from build123d import *

# Parameters (mm, degrees)
SKETCH_1_W      = 2
SKETCH_1_H      = 5
EXTRUDE_1_DEPTH = 2
FILLET_1_R      = 10


with BuildPart() as part:
    # 草图1 → 凸台-拉伸1 (new body)
    with BuildSketch(Plane(origin=(0, 0, 0), x_dir=(1, 0, 0), z_dir=(0, 1, 0))):
        with BuildLine():
            Line((10, 0), (0, 0))
            Line((0, 0), (0, -5))
            Line((0, -5), (0, -13.5))
            ThreePointArc((0, -13.5), (1.060660172, -13.939339828), (1.5, -15))
            ThreePointArc((1.5, -15), (1.060660172, -16.060660172), (0, -16.5))
            Line((0, -16.5), (0, -43.5))
            ThreePointArc((0, -43.5), (1.060660172, -43.939339828), (1.5, -45))
            ThreePointArc((1.5, -45), (1.060660172, -46.060660172), (0, -46.5))
            Line((0, -46.5), (0, -73.5))
            ThreePointArc((0, -73.5), (1.060660172, -73.939339828), (1.5, -75))
            Line((1.5, -75), (2.5, -75))
            Line((2.5, -75), (2.5, -72.5))
            Line((2.5, -72.5), (7.5, -72.5))
            Line((7.5, -72.5), (7.5, -75))
            Line((7.5, -75), (8.5, -75))
            ThreePointArc((8.5, -75), (8.939339828, -73.939339828), (10, -73.5))
            Line((10, -73.5), (10, -46.5))
            ThreePointArc((10, -46.5), (8.5, -45), (10, -43.5))
            Line((10, -43.5), (10, -16.5))
            ThreePointArc((10, -16.5), (8.5, -15), (10, -13.5))
            Line((10, -13.5), (10, -5))
            Line((10, -5), (10, 0))
        make_face()
        Polygon((2.5, -72.5), (2.5, -75), (5, -75), (7.5, -75), (7.5, -72.5), align=None)
        Polygon((5, -75), (2.5, -75), (2.5, -77.5), (7.5, -77.5), (7.5, -75), align=None)
        with BuildLine():
            Line((2.5, -75), (1.5, -75))
            ThreePointArc((1.5, -75), (1.060660172, -76.060660172), (0, -76.5))
            Line((0, -76.5), (0, -103.5))
            ThreePointArc((0, -103.5), (1.060660172, -103.939339828), (1.5, -105))
            ThreePointArc((1.5, -105), (1.060660172, -106.060660172), (0, -106.5))
            Line((0, -106.5), (0, -133.5))
            ThreePointArc((0, -133.5), (1.060660172, -133.939339828), (1.5, -135))
            ThreePointArc((1.5, -135), (1.060660172, -136.060660172), (0, -136.5))
            Line((0, -136.5), (0, -145))
            Line((0, -145), (0, -150))
            Line((0, -150), (10, -150))
            Line((10, -150), (10, -145))
            Line((10, -145), (10, -136.5))
            ThreePointArc((10, -136.5), (8.5, -135), (10, -133.5))
            Line((10, -133.5), (10, -106.5))
            ThreePointArc((10, -106.5), (8.5, -105), (10, -103.5))
            Line((10, -103.5), (10, -76.5))
            ThreePointArc((10, -76.5), (8.939339828, -76.060660172), (8.5, -75))
            Line((8.5, -75), (7.5, -75))
            Line((7.5, -75), (7.5, -77.5))
            Line((7.5, -77.5), (2.5, -77.5))
            Line((2.5, -77.5), (2.5, -75))
        make_face()
        with Locations((11, -147.5)):
            Rectangle(SKETCH_1_W, SKETCH_1_H)
        with Locations((-1, -147.5)):
            Rectangle(SKETCH_1_W, SKETCH_1_H)
        with Locations((11, -2.5)):
            Rectangle(SKETCH_1_W, SKETCH_1_H)
        with Locations((-1, -2.5)):
            Rectangle(SKETCH_1_W, SKETCH_1_H)
    extrude(amount=EXTRUDE_1_DEPTH)

    # 圆角1
    # the kernel refuses this fillet: 10 mm, written as the material it adds along each edge
    with BuildSketch(Plane(origin=(10, 0, 145), x_dir=(0, 0, -1), z_dir=(0, 1, 0)), Plane(origin=(0, 0, 5), x_dir=(0, 0, 1), z_dir=(0, 1, 0))) as fillet_1_piece_1:
        with BuildLine():
            CenterArc((6, -10), FILLET_1_R, 90, 36.869897646)
            Line((0, -2), (0, 0))
            Line((0, 0), (6, 0))
        make_face()
    extrude(amount=2)
    with BuildSketch(Plane(origin=(0, 0, 145), x_dir=(-1, 0, 0), z_dir=(0, 1, 0)), Plane(origin=(10, 0, 5), x_dir=(1, 0, 0), z_dir=(0, 1, 0))) as fillet_1_piece_2:
        with BuildLine():
            CenterArc((10, -6), FILLET_1_R, 143.130102354, 36.869897646)
            Line((0, -6), (0, 0))
            Line((0, 0), (2, 0))
        make_face()
    extrude(amount=2)


solid = part.part
Source: CAD feature listing. Evaluate the final solid. Frame: model axes, mm. Give positions to 0.01 mm unless a question says otherwise; leave off trailing zeros. Order: outer loops, then holes, each group sorted by start corner. A loop starts at its lowest first (then second) coordinate and runs counter-clockwise, first axis right, second up. Notation, with made-up numbers: (22, 89.25) -> (42, 89.25) arc R22 cw to (42, 109.25) -> close; hole circle Ø8 at (-36.75, 30). An arc over 180 degrees is marked (long way). Write item = value, one per line.
Item 1: Section query A-A (z = 95.5). Output: boundary loops of the cut face in (x, y).
Check result:
outline = (0, 0) -> (10, 0) -> (10, 2) -> (0, 2) -> close
Item 2: Ray query, probe 1 along Z at (x, y) = (0.5, 0.3); probe 2 along X at (y, z) = (0.45, 57.5); probe 3 along X at (y, z) = (0.75, 7.5). Return the intervals inside material, ascending.
Check result:
probe_1 = 0 to 13.59, 16.41 to 43.59, 46.41 to 73.59, 76.41 to 103.59, 106.41 to 133.59, 136.41 to 150
probe_2 = 0 to 10
probe_3 = -0.63 to 10.63
Item 3: Contact query for flat-ended pins moving along their axis: pin 1 (1 mm diameter, centred on y = 1.5, z = 109, fed in from -X); pin 2 (0.6 mm diameter, centred on y = 0.5, z = 31, fed in from +X); pin 3 (4 mm diameter, centred on x = 7, z = 98.5, fed in from -Y). Output: stop coordinate, or through.
Check result:
pin_1 = 0
pin_2 = 10
pin_3 = 0
Item 4: Section query B-B (z = 9.5). Output: boundary loops of the cut face in (x, y), then the cut area to 3 significant figures.
Check result:
outline = (-0.11, 0) -> (10.11, 0) -> (10.11, 2) -> (-0.11, 2) -> close
area = 20.5 mm²
